Here's how the part is built. I have some questions about the finished solid (model axes, mm). A direction names the side the tool comes from. Give positions to 0.01 mm unless a question says otherwise; leave off trailing zeros. Write each loop counter-clockwise with the first axis right and the second up, starting at its lowest first coordinate (ties: lowest second). Pieces come first, ordered by that corner, then holes. Notation, with made-up numbers: (75, -7.75) - (120, -7.75) arc R23 cw to (120, 3.25) - close; hole circle Ø11 at (79.5, 86.25). An arc over 180 degrees is marked (long way). One line per item, written item: value. Start each with the question number.
1) Imagine slicing it at D-D on z = 4.25. Write out the boundary of the cut face in (x, y).
2) Imagine slicing it at B-B on x = 4.75. Write out the boundary of the cut face in (y, z), plus the area to 3 significant figures.
3) Please list where these lines run through material, in increasing order: L1, parallel to Z at x = -3.25, y = -2.25; L2, parallel to Z at x = 1.5, y = -8.25; L3, parallel to Y at x = 0.75, z = -4. Write a range as [from, to].
4) Imagine slicing it at C-C on y = -5.75. Write out the boundary of the cut face in (x, z).
5) I'm going to push flat-ended pins straight in: P1, Ø1, axis at x = -3, z = -3, coming from the +Y side; P2, Ø1.5, axis at y = -8, z = 0.5, coming from the +X side; P3, Ø3, axis at x = 0.5, z = -3.5, coming from the -Y side. Where does each tip first touch, or does it pass through?
6) On a 3-axis mill with a long thin cutter (end or side, diameter ignored), from which of +Z, -Z, +X, -X, +Y, -Y can I reach the whole of each face in a straight line? I mean faces 4 (the flat face through (-3.54, -4.69, -2.59)), 5 (the cylindrical face through (2.15, -8.258, -3.547)), 6 (the flat face through (1.59, -2.96, -4.19)), 7 (the cylindrical face through (-1.793, -5.07, 3.554)), 8 (the flat face through (1.34, -4.93, 4.177)). Say none if no direction works.
7) Imagine slicing it at A-A on y = -9. Write out the boundary of the cut face in (x, z).
8) We'd pull the mould along X, two halves only. Please class faces 1 (the flat face through (4.62, -4.93, 1.25)), 2 (the cylindrical face through (-2.81, -8.26, -3.02)), 3 (the flat face through (0.54, -5.35, -4.36)): +X half, -X half, draft (parallel to the pull), parting line (faces both ways), or undercut.
from build123d import *

# Parameters (mm, degrees)
F1_DEPTH = 10
F2_R     = 4
F3_R     = 5
F4_R     = 5
F6_DEPTH = 10
F7_SIZE  = 1.5
F8_R     = 3


with BuildPart() as f1:
    # F0 (on Front) → F1 (new body)
    with BuildSketch(Plane.XZ):
        Polygon((4.8367500103, 1.0255116078), (0.5193184536, 4.9169231297), (-4.515793555, 2.0133140065), (-3.3102323568, -3.6726266437), (2.4699574478, -4.2831221003), align=None)
    extrude(amount=F1_DEPTH)

    # F2
    f2_edges = [f1.edges().sort_by_distance(p)[0] for p in [
        (-0.420137, -10, -3.977874),
    ]]
    fillet(f2_edges, radius=F2_R)

    # F3
    f3_edges = [f1.edges().sort_by_distance(p)[0] for p in [
        (4.83675, -5, 1.025512),
    ]]
    fillet(f3_edges, radius=F3_R)

    # F4
    f4_edges = [f1.edges().sort_by_distance(p)[0] for p in [
        (-4.515794, -5, 2.013314),
    ]]
    fillet(f4_edges, radius=F4_R)

    # F5 (on Front) → F6 (join)
    with BuildSketch(Plane.XZ):
        Polygon((5.4859916503, 2.4391776778), (-4.8553856584, 3.5314192952), (-0.6306059919, -5.970596973), align=None)
    extrude(amount=F6_DEPTH)

    # F7
    f7_edges = [f1.edges().sort_by_distance(p)[0] for p in [
        (-0.630606, -5, -5.970597),
    ]]
    chamfer(f7_edges, length=F7_SIZE)

    # F8
    f8_edges = [f1.edges().sort_by_distance(p)[0] for p in [
        (-0.494162, -10, -4.678744),
    ]]
    fillet(f8_edges, radius=F8_R)


solid = f1.part
Numbers:
1. outline: (-0.64, -10) - (1.26, -10) - (1.26, 0) - (-0.64, 0) - close
2. outline: (-10, 1.43) - (0, 1.43) - (0, 2.52) - (-10, 2.52) - close
2. area: 10.9 mm^2
3. L1: [-3.68, 3.36]
3. L2: [-3.48, 4.03]
3. L3: [-9.05, 0]
4. outline: (-4.86, 3.53) - (-3.68, 0.88) arc R5 ccw to (-3.76, -1.54) - (-3.31, -3.67) - (-1.57, -3.86) - (-1.24, -4.6) - (0.25, -4.76) - (0.73, -4.1) - (2.47, -4.28) - (3.36, -2.29) arc R5 ccw to (3.78, 0.09) - (5.49, 2.44) - (2.81, 2.72) arc R5 ccw to (2.14, 3.46) - (0.52, 4.92) - (-1.37, 3.83) arc R5 ccw to (-2.18, 3.25) - close
5. P1: y = 0
5. P2: x = 4.62
5. P3: y = -9.99
6. face 4: -Z, -X, +Y, -Y
6. face 5: -Z, -Y
6. face 6: -Z, +Y, -Y
6. face 7: +Z, +Y, -Y
6. face 8: +Z, +X, +Y, -Y
7. outline: (-4.86, 3.53) - (-3.68, 0.88) arc R5 ccw to (-3.76, -1.54) - (-3.61, -2.28) - (-2.21, -2.43) - (-1.6, -3.79) - (0.77, -4.04) - (1.65, -2.83) - (3.05, -2.98) - (3.36, -2.29) arc R5 ccw to (3.78, 0.09) - (5.49, 2.44) - (2.81, 2.72) arc R5 ccw to (2.14, 3.46) - (0.52, 4.92) - (-1.37, 3.83) arc R5 ccw to (-2.18, 3.25) - close
8. face 1: +X half
8. face 2: -X half
8. face 3: undercut
